Can you work these out from the model? Positions are in its coordinate system, mm. Coordinates: 2 decimals unless noted, no trailing zeros. Order: outer loops, then holes, each group sorted by start corner. A loop starts at its lowest first (then second) coordinate and runs counter-clockwise, first axis right, second up. Notation, with made-up numbers: (2.5, 1.25) -> (39.5, 1.25) arc R35 ccw to (39.5, 37.25) -> close; hole circle Ø5 at (87.5, 78). An arc over 180 degrees is marked (long way). Answer in a Markdown table with one row per item.
```python
from build123d import *

# Parameters (mm, degrees)
SKETCH1_R           = 4.82
SKETCH1_R_2         = 3.175
SKETCH1_W           = 20
SKETCH1_H           = 70
BOSS_EXTRUDE1_DEPTH = 3.175


with BuildPart() as part:
    # Sketch1 → Boss-Extrude1 (new body)
    with BuildSketch(Plane(origin=(0, 0, 0), x_dir=(1, 0, 0), z_dir=(0, 1, 0))):
        with BuildLine():
            ThreePointArc((50, -25), (25, 0), (0, -25))
            Line((0, -25), (0, -274.999999959))
            ThreePointArc((0, -274.999999959), (24.999999979, -300), (50, -275))
            Line((50, -275), (50, -25))
        make_face()
        with Locations(Location((25, -25, 0), (0, 0, 270))):
            Circle(SKETCH1_R, mode=Mode.SUBTRACT)
        with Locations(Location((25, -95, 0), (0, 0, 270))):
            Circle(SKETCH1_R_2, mode=Mode.SUBTRACT)
        with Locations(Location((25, -205, 0), (0, 0, 270))):
            Circle(SKETCH1_R_2, mode=Mode.SUBTRACT)
        with Locations((25, -150)):
            Rectangle(SKETCH1_W, SKETCH1_H, mode=Mode.SUBTRACT)
        with Locations(Location((25, -275, 0), (0, 0, 270))):
            Circle(SKETCH1_R, mode=Mode.SUBTRACT)
    extrude(amount=BOSS_EXTRUDE1_DEPTH)


solid = part.part
```
(1) Will this pin go through, and if not, where does the flat tip stop? pin 1 Ø1.6 at (x, y) = (23, 1.5) entering from +Z.
Response values:
| item | result |
|---|---|
| pin 1 | z = 299.97 |
(2) Suppose I cut it at C-C (y = 0.85). Please give me the cut outline in (x, z) (3 decimals), and give its area (3 significant figures).
Response values:
| item | result |
|---|---|
| outline | (0, 25) arc R25 ccw to (50, 25) -> (50, 275) arc R25 ccw to (0, 275) -> close; hole (15, 115) -> (35, 115) -> (35, 185) -> (15, 185) -> close; hole circle Ø9.64 at (25, 25); hole circle Ø9.64 at (25, 275); hole circle Ø6.35 at (25, 95); hole circle Ø6.35 at (25, 205) |
| area | 12,900 mm2 |
(3) Suppose I cut it at B-B (x = 25). Please give me the cut outline in (y, z) (3 decimals), and give its area (3 significant figures).
Response values:
| item | result |
|---|---|
| outline | (0, 0) -> (3.175, 0) -> (3.175, 20.18) -> (0, 20.18) -> close; (0, 29.82) -> (3.175, 29.82) -> (3.175, 91.825) -> (0, 91.825) -> close; (0, 98.175) -> (3.175, 98.175) -> (3.175, 115) -> (0, 115) -> close; (0, 185) -> (3.175, 185) -> (3.175, 201.825) -> (0, 201.825) -> close; (0, 208.175) -> (3.175, 208.175) -> (3.175, 270.18) -> (0, 270.18) -> close; (0, 279.82) -> (3.175, 279.82) -> (3.175, 300) -> (0, 300) -> close |
| area | 629 mm2 |
(4) I need wall thicknesses on line 1 (X direction, y = 2.65, z = 117); line 2 (Z direction, x = 24.5, y = 0.25) (3 decimals); line 3 (X direction, y = 1.7, z = 205) (3 decimals). Which ranges of each line are inside material? Lowest first, please. Write a range as [from, to].
Response values:
| item | result |
|---|---|
| line 1 | [0, 15], [35, 50] |
| line 2 | [0.005, 20.206], [29.794, 91.865], [98.135, 115], [185, 201.865], [208.135, 270.206], [279.794, 299.995] |
| line 3 | [0, 21.825], [28.175, 50] |
(5) We'd pull the mould along X, two halves only. Please class faces 1 (the cylindrical face through (25.55, 1.565, 0.006)), 2 (the cylindrical face through (22.067, 1.565, 21.175)), 3 (the cylindrical face through (26.448, 1.565, 279.597)), 4 (the flat face through (14, 0, 148)): +X half, -X half, draft (parallel to the pull), parting line (faces both ways), or undercut.
Response values:
| item | result |
|---|---|
| face 1 | parting line |
| face 2 | undercut |
| face 3 | undercut |
| face 4 | draft |
(6) Suppose I cut it at D-D (z = 122.5). Please give me the cut outline in (x, y) (3 decimals).
Response values:
| item | result |
|---|---|
| outline | (0, 0) -> (15, 0) -> (15, 3.175) -> (0, 3.175) -> close; (35, 0) -> (50, 0) -> (50, 3.175) -> (35, 3.175) -> close |
(7) Suppose I cut it at A-A (z = 205). Please give me the cut outline in (x, y) (3 decimals), and give its area (3 significant figures).
Response values:
| item | result |
|---|---|
| outline | (0, 0) -> (21.825, 0) -> (21.825, 3.175) -> (0, 3.175) -> close; (28.175, 0) -> (50, 0) -> (50, 3.175) -> (28.175, 3.175) -> close |
| area | 139 mm2 |
